Design review of the part built by this model. Coordinates are the model's own, in mm. Round coordinates to 2 decimals unless told otherwise and drop trailing zeros. Write each loop counter-clockwise with the first axis right and the second up, starting at its lowest first coordinate (ties: lowest second). Pieces come first, ordered by that corner, then holes. Notation, with made-up numbers: M 59.5,-25.5 L 76.5,-25.5 A10 cw 76.5,-19.5 Z; hole C 15.5,1.5 d11. An arc over 180 degrees is marked long. Use CSV: the item, a comma, the result in double quotes.
from build123d import *

# Parameters (mm, degrees)
F0_R     = 16
F1_DEPTH = 9
F2_R     = 7.5
F3_DEPTH = 9.001
F4_SIZE  = 0.5


with BuildPart() as f1:
    # F0 (on Right) → F1 (new body)
    with BuildSketch(Plane.YZ):
        Circle(F0_R)
    extrude(amount=-F1_DEPTH)

    # F2 (on face) → F3 (cut, through all)
    with BuildSketch(Plane.YZ):
        Circle(F2_R)
    extrude(amount=-F3_DEPTH, mode=Mode.SUBTRACT)

    # F4
    f4_edges = [f1.edges().sort_by_distance(p)[0] for p in [
        (-4.5, 16, 0),
        (0, -16, 0),
        (-9, -16, 0),
    ]]
    chamfer(f4_edges, length=F4_SIZE)


solid = f1.part
1) For pin 1 Ø2 at (x, y) = (-3, 4) entering from +Z; pin 2 Ø4 at (x, y) = (-7.5, -8.5) entering from +Z; pin 3 Ø10 at (y, z) = (-0.5, 12) entering from +X; pin 4 Ø1 at (x, z) = (-6.5, 3.5) entering from -Y, all flat-tipped, find the tip position at first contact; note any pin that passes through.
Answers:
pin 1,"z = 15.72"
pin 2,"z = 14.62"
pin 3,"x = 0"
pin 4,"y = -15.72"
2) Add section A-A on z = 0. Write out the cut boundary in (x, y), then the cut area to 4 significant figures.
Answers:
outline,"M -9,-15.5 L -8.5,-16 L -0.5,-16 L 0,-15.5 L 0,-7.5 L -9,-7.5 Z; M -9,7.5 L 0,7.5 L 0,15.5 L -0.5,16 L -8.5,16 L -9,15.5 Z"
area,"152.5 mm²"
3) Add section C-C on x = -7.5. Write out the cut boundary in (y, z).
Answers:
outline,"C 0,0 d32; hole C 0,0 d15"
4) Wall thickness on line 1 along Z through (x, y) = (-3, 0); line 2 along Y through (x, z) = (-7.25, -2); line 3 along Y through (x, z) = (-7.75, -4): over which ranges is each line inside the solid? List them lowest first. Write a range as [from, to].
Answers:
line 1,"[-16, -7.5], [7.5, 16]"
line 2,"[-15.87, -7.23], [7.23, 15.87]"
line 3,"[-15.49, -6.34], [6.34, 15.49]"
5) The part is to be moulded in two halves that separate along Y. For faces 1 (the face through (-9, 7, 4)), 2 (the face through (-4.44, -3.47, -15.62)), 3 (the face through (-4.437, -7.493, 0.33)), say which applies: released by +Y, released by -Y, zero draft, split by the parting line, or undercut.
Answers:
face 1,"zero draft"
face 2,"split by the parting line"
face 3,"undercut"
